Geometry check sheet. Reference: the model listing, model coordinates, mm. Face numbers are marked on the shaded views. A direction names the side the tool comes from. Coordinates: 2 decimals unless noted, no trailing zeros. Loops run counter-clockwise (first coordinate to the right, second up) from the corner with the lowest first, then second, coordinate; pieces in that order, holes last. Notation, with made-up numbers: M 19,57 L 40,57 A23 ccw 40,86 Z; hole C 81.25,16 d3. An arc over 180 degrees is marked long. Use CSV: the item, a comma, the result in double quotes.
```python
from build123d import *

# Parameters (mm, degrees)
F0_W     = 10.4597713798
F0_H     = 24
F0_W_2   = 10
F0_H_2   = 5
F1_DEPTH = 1
F2_DEPTH = 3
F3_DEPTH = 25
F4_DEPTH = 25
F5_SIZE  = 5
F6_R     = 2
F7_DEPTH = 25
F6_R_2   = 3.5
F8_DEPTH = 2


with BuildPart() as f1:
    # F0 (on Top) → F1 (new body)
    with BuildSketch(Plane.XY):
        Rectangle(F0_W, F0_H)
        Rectangle(F0_W_2, F0_H_2, mode=Mode.SUBTRACT)
        Rectangle(F0_W_2, F0_H_2)
    extrude(amount=F1_DEPTH)

    # F0 (on Top) → F2 (join)
    with BuildSketch(Plane.XY):
        Rectangle(F0_W, F0_H)
        Rectangle(F0_W_2, F0_H_2, mode=Mode.SUBTRACT)
    extrude(amount=F2_DEPTH)

    # F3 (cut): a face of the model
    f3_faces = [f1.faces().sort_by_distance(p)[0] for p in [
        (-5, 0, 2),
    ]]
    extrude(f3_faces, amount=-F3_DEPTH, mode=Mode.SUBTRACT)

    # F4 (cut): a face of the model
    f4_faces = [f1.faces().sort_by_distance(p)[0] for p in [
        (5, 0, 2),
    ]]
    extrude(f4_faces, amount=-F4_DEPTH, mode=Mode.SUBTRACT)

    # F5
    f5_edges = [f1.edges().sort_by_distance(p)[0] for p in [
        (-5.229886, -12, 1.5),
        (5.229886, -12, 1.5),
        (5.229886, 12, 1.5),
        (-5.229886, 12, 1.5),
    ]]
    chamfer(f5_edges, length=F5_SIZE)

    # F6 (on face) → F7 (cut)
    with BuildSketch(Plane(origin=(0, 0, 0), x_dir=(1, 0, 0), z_dir=(0, 0, -1))):
        with BuildLine():
            ThreePointArc((2, 6.5), (1.4142135624, 7.9142135624), (0, 8.5))
            ThreePointArc((0, 8.5), (-1.4142135624, 5.0857864376), (2, 6.5))
        make_face()
        with Locations((0, -6.5)):
            Circle(F6_R)
    extrude(amount=-F7_DEPTH, mode=Mode.SUBTRACT)

    # F6 (on face) → F8 (join)
    with BuildSketch(Plane(origin=(0, 0, 0), x_dir=(1, 0, 0), z_dir=(0, 0, -1))):
        with BuildLine():
            ThreePointArc((2.4209805773, 9.8089051126), (1.2734773336, 10.3972112441), (0, 10.6))
            ThreePointArc((0, 10.6), (-1.2734773336, 10.3972112441), (-2.4209805773, 9.8089051126))
            Line((-2.4209805773, 9.8089051126), (-3.3089051126, 8.9209805773))
            ThreePointArc((-3.3089051126, 8.9209805773), (-1.2734773336, 2.6027887559), (4.1, 6.5))
            ThreePointArc((4.1, 6.5), (3.8972112441, 7.7734773336), (3.3089051126, 8.9209805773))
            Line((3.3089051126, 8.9209805773), (2.4209805773, 9.8089051126))
        make_face()
        with BuildLine():
            ThreePointArc((3.5, 6.5), (-2.4748737342, 4.0251262658), (0, 10))
            ThreePointArc((0, 10), (2.4748737342, 8.9748737342), (3.5, 6.5))
        make_face(mode=Mode.SUBTRACT)
        with BuildLine():
            Line((2.4209805773, -9.8089051126), (3.3089051126, -8.9209805773))
            ThreePointArc((3.3089051126, -8.9209805773), (3.8972112441, -7.7734773336), (4.1, -6.5))
            ThreePointArc((4.1, -6.5), (-1.2734773336, -2.6027887559), (-3.3089051126, -8.9209805773))
            Line((-3.3089051126, -8.9209805773), (-2.4209805773, -9.8089051126))
            ThreePointArc((-2.4209805773, -9.8089051126), (0, -10.6), (2.4209805773, -9.8089051126))
        make_face()
        with Locations((0, -6.5)):
            Circle(F6_R_2, mode=Mode.SUBTRACT)
    extrude(amount=F8_DEPTH)


solid = f1.part
```
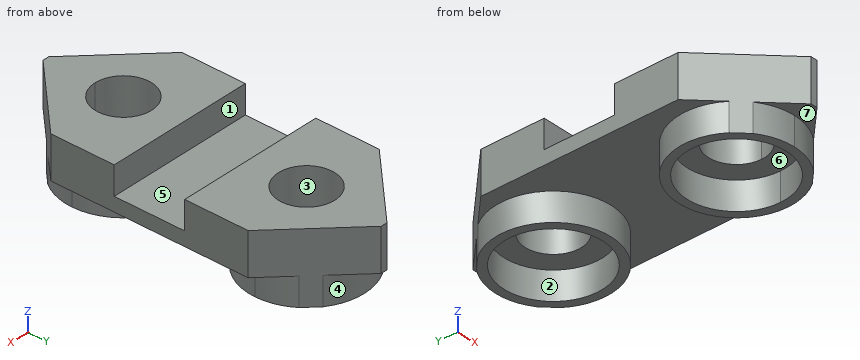
1. Thickness scan on line 1 (Y direction, x = 0, z = 0.85); line 2 (X direction, y = -6.5, z = -0.4); line 3 (X direction, y = -6.5, z = 0.8). Record the ranges inside material, lowest first. Write a range as [from, to].
The answers:
line 1,"[-12, -8.5], [-4.5, 4.5], [8.5, 12]"
line 2,"[-4.1, -3.5], [3.5, 4.1]"
line 3,"[-5.23, -2], [2, 5.23]"
2. Section check A-A, the plane z = 1.6. Record the cut outline in (x, y).
The answers:
outline,"M -5.23,-7 L -0.23,-12 L 0.23,-12 L 5.23,-7 L 5.23,-2.5 L -5.23,-2.5 Z; M -5.23,2.5 L 5.23,2.5 L 5.23,7 L 0.23,12 L -0.23,12 L -5.23,7 Z; hole C 0,-6.5 d4; hole C 0,6.5 d4"
3. Section check B-B, the plane y = 5. Record the cut outline in (x, z).
The answers:
outline,"M -5.23,0 L -3.82,0 L -3.82,-2 L -3.16,-2 L -3.16,0 L -1.32,0 L -1.32,3 L -5.23,3 Z; M 1.32,0 L 3.16,0 L 3.16,-2 L 3.82,-2 L 3.82,0 L 5.23,0 L 5.23,3 L 1.32,3 Z"
4. Release check for a two-part mould opening along Y. For the marked faces 4, 5, 6 and 7 record: +Y half, -Y half, draft (parallel to the pull), parting line (faces both ways), or undercut.
The answers:
face 4,"+Y half"
face 5,"undercut"
face 6,"undercut"
face 7,"draft"
5. Set-up check for the marked faces 1, 2 and 3: record each of +Z, -Z, +X, -X, +Y, -Y from which the full face is reachable in a straight line by a thin tool's end or side.
The answers:
face 1,"+Z, +X, -X"
face 2,"-Z"
face 3,"+Z, -Z"
6. Gauge pin test, flat ends, axial feed: P1, Ø1.6, axis at x = 2, z = 2.5, coming from the +Y side; P2, Ø1, axis at x = 0.5, y = -7.5, coming from the +Z side; P3, Ø1, axis at x = -3.5, z = -0.5, coming from the +Y side; P4, Ø1.5, axis at x = -0.5, y = 1, coming from the +Z side. Record the tip position at first contact, or that the pin passes through.
The answers:
P1,"y = 11.03"
P2,"through"
P3,"y = 9.23"
P4,"z = 1"
7. Section check D-D, the plane z = -1.4. Record the cut outline in (x, y), plus the area to 3 significant figures.
The answers:
outline,"M -3.31,-8.92 L -2.42,-9.81 A4.1 ccw 2.42,-9.81 L 3.31,-8.92 A4.1 ccw long Z; M -3.31,8.92 A4.1 ccw long 3.31,8.92 L 2.42,9.81 A4.1 ccw -2.42,9.81 Z; hole C 0,-6.5 d7; hole C 0,6.5 d7"
area,"28.5 mm^2"
8. Section check C-C, the plane x = -1.25. Count the separate pieces of the cut face and the enclosed holes in it, plus the area to 3 significant figures.
The answers:
separate pieces,"3"
enclosed holes,"0"
area,"42.2 mm^2"
